Source: three-view drawing plus pictorial views. Frame: mm from the lowest corner of the part. Round coordinates to 2 decimals unless told otherwise and drop trailing zeros. Loops run counter-clockwise (first coordinate to the right, second up) from the corner with the lowest first, then second, coordinate; pieces in that order, holes last. Notation, with made-up numbers: (65.25, 50) -> (93.25, 50) arc R20 ccw to (93.25, 78) -> close; hole circle Ø4 at (59, -21). An arc over 180 degrees is marked (long way). Put each result on its own line as item: value. Start each with the question number.
1. Draft query along Z for the marked faces 1, 2 and 3. Return one class per face: pulls with the +Z half, pulls with the -Z half, needs draft (parallel to the pull), parting line crosses it, or undercut.
2. Cut plane A-A (y = 48). Return the cut outline in (x, z), then the cut area to 3 significant figures.
3. Contact query for flat-ended pins moving along their axis: pin 1 (6 mm diameter, centred on x = 34.5, y = 69.5, fed in from -Z); pin 2 (12 mm diameter, centred on x = 23.5, y = 13, fed in from -Z); pin 3 (4 mm diameter, centred on x = 61.5, y = 56, fed in from +Z); pin 4 (1 mm diameter, centred on x = 73.5, z = 88, fed in from +Y). Output: stop coordinate, or through.
4. Material intervals for L1, parallel to X at y = 121, z = 57.5; L2, parallel to Z at x = 45, y = 70.5; L3, parallel to X at y = 60.5, z = 38 (1 decimal), sorted ascending.
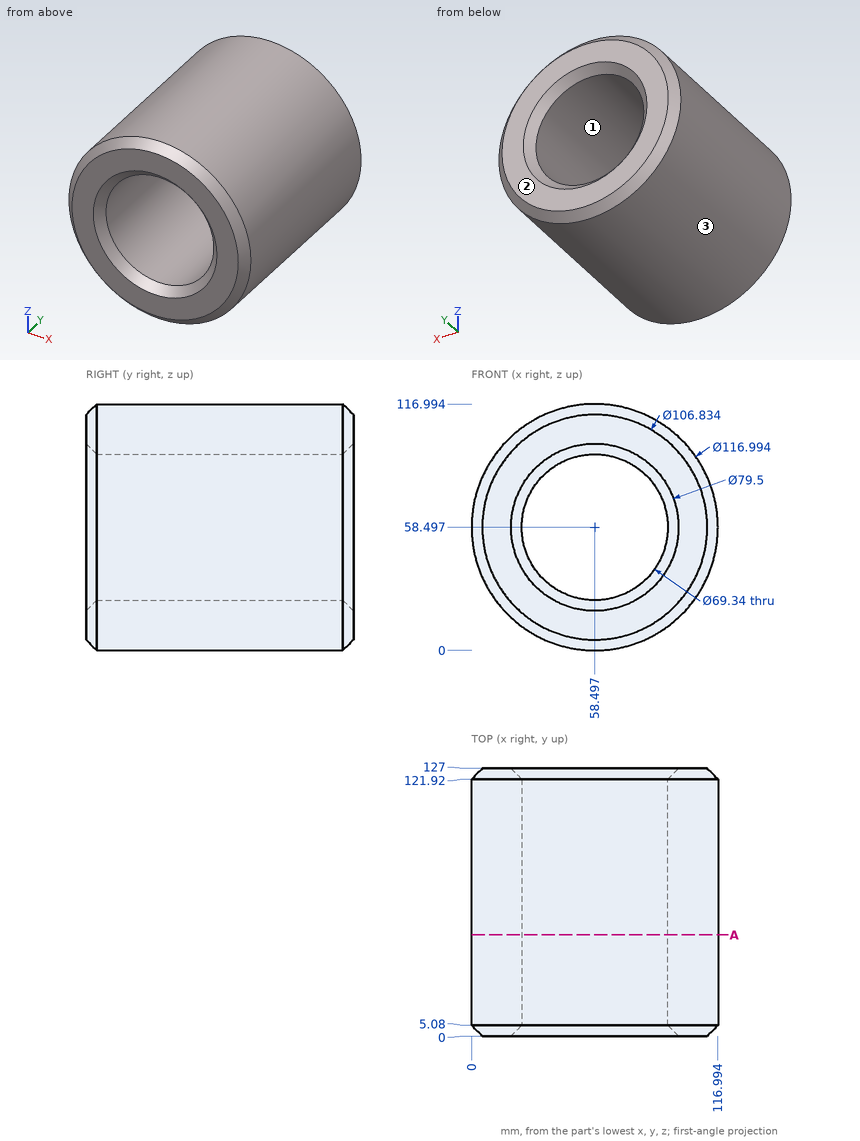
Solution:
1. face 1: undercut
1. face 2: needs draft
1. face 3: parting line crosses it
2. outline: circle Ø116.99 at (58.5, 58.5); hole circle Ø69.34 at (58.5, 58.5)
2. area: 6,970 mm^2
3. pin 1: stops at z = 3.9
3. pin 2: stops at z = 7.69
3. pin 3: stops at z = 116.99
3. pin 4: passes through
4. L1: x = 0.01 to 23.84, 93.15 to 116.99
4. L2: z = 1.58 to 26.56, 90.43 to 115.42
4. L3: x = 3.7 to 30.5, 86.5 to 113.3
